Check sheet for the modelled part. Datum: model origin and axes. Units: mm. Round coordinates to 2 decimals unless told otherwise and drop trailing zeros. Loops run counter-clockwise (first coordinate to the right, second up) from the corner with the lowest first, then second, coordinate; pieces in that order, holes last. Notation, with made-up numbers: (16.25, 33) -> (49.25, 33) arc R25 ccw to (49.25, 50) -> close; hole circle Ø7 at (67, 19). An arc over 180 degrees is marked (long way). Use one line per item in the form item = value. Start each with the question number.
(1) Go/stop test with a flat-tipped pin: pin 1 (3.5 mm diameter, centred on x = 398.24, z = 35.45, fed in from +Y). Record where the tip stops, or that it passes through.
(2) Sectioned sample at D-D (x = 373). Record the cut outline in (y, z) (3 decimals).
(3) Material ranges on probe 1 along X at (y, z) = (61.5, 182); probe 2 along X at (y, z) = (63.75, 152); probe 3 along X at (y, z) = (62.75, 56.5), recorded low to high. Write a range as [from, to].
(4) Sectioned sample at C-C (y = 65). State how many separate pieces and enclosed holes the cut face has, and give its area (3 significant figures).
(5) Sectioned sample at A-A (x = 99). Record the cut outline in (y, z) (3 decimals).
(6) Sectioned sample at B-B (z = 127). Record the cut outline in (x, y), and give its area (3 significant figures).
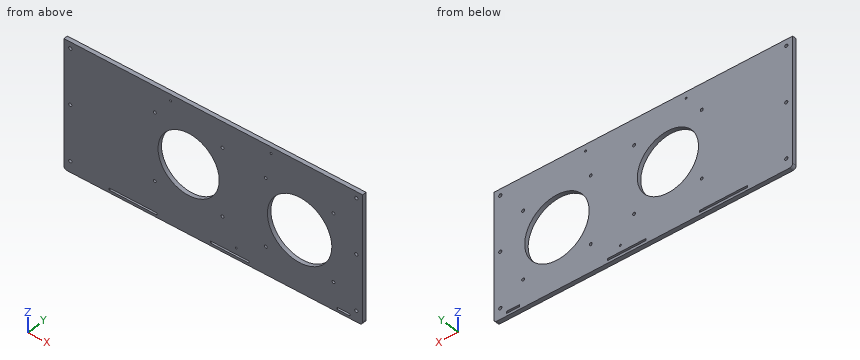
from build123d import *

# Parameters (mm, degrees)
SKETCH1_W           = 463.88
SKETCH1_H           = 192
BOSS_EXTRUDE1_DEPTH = 6.35
SKETCH4_R           = 2.5
CUT_EXTRUDE2_DEPTH  = 484.483469107
SKETCH2_W           = 463.88
SKETCH2_H           = 7.175
BOSS_EXTRUDE2_DEPTH = 6.35
SKETCH3_W           = 74.25
SKETCH3_H           = 3.175
SKETCH3_W_2         = 59.87
SKETCH3_W_3         = 20
CUT_EXTRUDE1_DEPTH  = 484.483469107
SKETCH5_R           = 1.5
CUT_EXTRUDE3_DEPTH  = 484.483469107
FILLET1_R           = 5
SKETCH6_R           = 47.5
SKETCH6_R_2         = 50
SKETCH6_R_3         = 2.25
CUT_EXTRUDE4_DEPTH  = 484.483469107


with BuildPart() as part:
    # Sketch1 → Boss-Extrude1 (new body)
    with BuildSketch(Plane(origin=(0, 60, 0), x_dir=(1, 0, 0), z_dir=(0, 1, 0))):
        with Locations((211.74, -96)):
            Rectangle(SKETCH1_W, SKETCH1_H)
    extrude(amount=BOSS_EXTRUDE1_DEPTH)

    # Sketch4 → Cut-Extrude2 (cut, through all)
    with BuildSketch(Plane(origin=(0, 66.35, 0), x_dir=(1, 0, 0), z_dir=(0, 1, 0))):
        with Locations(Location((433.68, -10, 0), (0, 0, 270))):
            Circle(SKETCH4_R)
        with Locations(Location((433.68, -96, 0), (0, 0, 270))):
            Circle(SKETCH4_R)
        with Locations(Location((433.68, -182, 0), (0, 0, 270))):
            Circle(SKETCH4_R)
        with Locations(Location((-10.2, -182, 0), (0, 0, 270))):
            Circle(SKETCH4_R)
        with Locations(Location((-10.2, -96, 0), (0, 0, 270))):
            Circle(SKETCH4_R)
        with Locations(Location((-10.2, -10, 0), (0, 0, 270))):
            Circle(SKETCH4_R)
    extrude(amount=-CUT_EXTRUDE2_DEPTH, mode=Mode.SUBTRACT)

    # Sketch2 → Boss-Extrude2 (add)
    with BuildSketch(Plane(origin=(0, 66.35, 0), x_dir=(1, 0, 0), z_dir=(0, 1, 0))):
        with Locations((211.74, 3.5875)):
            Rectangle(SKETCH2_W, SKETCH2_H)
    extrude(amount=-BOSS_EXTRUDE2_DEPTH)

    # Sketch3 → Cut-Extrude1 (cut, through all)
    with BuildSketch(Plane(origin=(0, 66.35, 0), x_dir=(1, 0, 0), z_dir=(0, 1, 0))):
        with Locations((87.375, 1.5875)):
            Rectangle(SKETCH3_W, SKETCH3_H)
        with Locations((237.435, 1.5875)):
            Rectangle(SKETCH3_W_2, SKETCH3_H)
        with Locations((413.68, 1.5875)):
            Rectangle(SKETCH3_W_3, SKETCH3_H)
    extrude(amount=-CUT_EXTRUDE1_DEPTH, mode=Mode.SUBTRACT)

    # Sketch5 → Cut-Extrude3 (cut, through all)
    with BuildSketch(Plane(origin=(0, 66.35, 0), x_dir=(1, 0, 0), z_dir=(0, 1, 0))):
        with Locations(Location((247.37, -10, 0), (0, 0, 270))):
            Circle(SKETCH5_R)
        with Locations(Location((145.287005384, -182, 0), (0, 0, 270))):
            Circle(SKETCH5_R)
        with Locations(Location((301.287005384, -182, 0), (0, 0, 270))):
            Circle(SKETCH5_R)
    extrude(amount=-CUT_EXTRUDE3_DEPTH, mode=Mode.SUBTRACT)

    # Fillet1
    fillet1_edges = [part.edges().sort_by_distance(p)[0] for p in [
        (-20.2, 63.175, -7.175),
        (443.68, 63.175, -7.175),
    ]]
    fillet(fillet1_edges, radius=FILLET1_R)

    # Sketch6 → Cut-Extrude4 (cut, through all)
    with BuildSketch(Plane(origin=(0, 66.35, 0), x_dir=(1, 0, 0), z_dir=(0, 1, 0))):
        with Locations(Location((173.5, -99.5, 0), (0, 0, 270))):
            Circle(SKETCH6_R)
        with Locations(Location((345.74, -87.95, 0), (0, 0, 270))):
            Circle(SKETCH6_R_2)
        with Locations(Location((121, -47, 0), (0, 0, 270))):
            Circle(SKETCH6_R_3)
        with Locations(Location((226, -47, 0), (0, 0, 270))):
            Circle(SKETCH6_R_3)
        with Locations(Location((226, -152, 0), (0, 0, 270))):
            Circle(SKETCH6_R_3)
        with Locations(Location((121, -152, 0), (0, 0, 270))):
            Circle(SKETCH6_R_3)
        with Locations(Location((293.24, -140.45, 0), (0, 0, 270))):
            Circle(SKETCH6_R_3)
        with Locations(Location((293.24, -35.45, 0), (0, 0, 270))):
            Circle(SKETCH6_R_3)
        with Locations(Location((398.24, -35.45, 0), (0, 0, 270))):
            Circle(SKETCH6_R_3)
        with Locations(Location((398.24, -140.45, 0), (0, 0, 270))):
            Circle(SKETCH6_R_3)
    extrude(amount=-CUT_EXTRUDE4_DEPTH, mode=Mode.SUBTRACT)


solid = part.part
Checks:
q1.pin_1 = through
q2.outline = (60, -7.175) -> (66.35, -7.175) -> (66.35, 46.035) -> (60, 46.035) -> close; (60, 129.865) -> (66.35, 129.865) -> (66.35, 192) -> (60, 192) -> close
q3.probe_1 = [-20.2, -12.7], [-7.7, 143.79], [146.79, 299.79], [302.79, 431.18], [436.18, 443.68]
q3.probe_2 = [-20.2, 118.75], [123.25, 223.75], [228.25, 443.68]
q3.probe_3 = [-20.2, 153.32], [193.68, 306.87], [384.61, 443.68]
q4.separate_pieces = 1
q4.enclosed_holes = 22
q4.area = 76,700 mm2
q5.outline = (60, -7.175) -> (66.35, -7.175) -> (66.35, -3.175) -> (60, -3.175) -> close; (60, 0) -> (66.35, 0) -> (66.35, 192) -> (60, 192) -> close
q6.outline = (-20.2, 60) -> (134.77, 60) -> (134.77, 66.35) -> (-20.2, 66.35) -> close; (212.23, 60) -> (314.51, 60) -> (314.51, 66.35) -> (212.23, 66.35) -> close; (376.97, 60) -> (443.68, 60) -> (443.68, 66.35) -> (376.97, 66.35) -> close
q6.area = 2,060 mm2
